Could you check a few things on this model? Use its own coordinates, in mm. A direction names the side the tool comes from. Round coordinates to 2 decimals unless told otherwise and drop trailing zeros. Loops run counter-clockwise (first coordinate to the right, second up) from the corner with the lowest first, then second, coordinate; pieces in that order, holes last. Notation, with made-up numbers: (-26.75, 51) - (-17.75, 51) arc R20 ccw to (-17.75, 67) - close; hole circle Ø8 at (56.25, -7.75). An arc over 180 degrees is marked (long way). Answer as CSV lines item,"result". Start each with the question number.
1) Which directions (+Z, -Z, +X, -X, +Y, -Y) give clear straight access to the entire face, cutting with the end or side of a thin tool? Please do faces 4 (the face through (-4.2, -2.7, -1)), 5 (the face through (0, 1, -6)), 6 (the face through (0, 1, 5)).
2) I'm going to push flat-ended pins straight in: pin 1 Ø6 at (x, z) = (-0.5, 0.5) entering from -Y; pin 2 Ø4 at (y, z) = (-3.5, -0.5) entering from -X; pin 3 Ø5 at (x, z) = (0.5, -3.5) entering from -Y. Where does each tip first touch, or does it pass through?
3) We'd pull the mould along Y, two halves only. Please class faces 1 (the face through (2.3, -2.7, -1)), 2 (the face through (0, 2, -1)), 3 (the face through (0, 0, -1)): pulls with the +Y half, pulls with the -Y half, needs draft (parallel to the pull), parting line crosses it, or undercut.
4) Please list where these lines run through material, in increasing order: line 1 along Z through (x, y) = (3.75, 1); line 2 along X through (y, z) = (0.5, 4.5); line 3 along Y through (x, z) = (-8, 5.5).
5) Suppose I cut it at D-D, the plane z = -1. Write out the boundary of the cut face in (x, y), then the cut area to 3 significant figures.
6) Suppose I cut it at B-B, the plane z = 4. Write out the boundary of the cut face in (x, y).
7) Suppose I cut it at C-C, the plane y = -3. Write out the boundary of the cut face in (x, z), then the cut area to 3 significant figures.
8) Suppose I cut it at A-A, the plane x = 3.25. Write out the boundary of the cut face in (y, z), then the cut area to 3 significant figures.
```python
from build123d import *

# Parameters (mm, degrees)
SKETCH1_W           = 19.9
SKETCH1_H           = 12
BOSS_EXTRUDE1_DEPTH = 2
SKETCH2_W           = 11.8
SKETCH2_H           = 5
CUT_EXTRUDE1_DEPTH  = 3
CHAMFER1_SIZE       = 1.25
SKETCH3_R           = 0.95
BOSS_EXTRUDE2_DEPTH = 5.6
CHAMFER2_SIZE       = 0.2


with BuildPart() as part:
    # Sketch1 → Boss-Extrude1 (new body)
    with BuildSketch(Plane(origin=(0, 0, 0), x_dir=(1, 0, 0), z_dir=(0, 1, 0))):
        Rectangle(SKETCH1_W, SKETCH1_H)
    extrude(amount=BOSS_EXTRUDE1_DEPTH)

    # Sketch2 → Cut-Extrude1 (cut, through all)
    with BuildSketch(Plane(origin=(0, 2, 0), x_dir=(1, 0, 0), z_dir=(0, 1, 0))):
        with Locations((0, -2.5)):
            Rectangle(SKETCH2_W, SKETCH2_H)
    extrude(amount=-CUT_EXTRUDE1_DEPTH, mode=Mode.SUBTRACT)

    # Chamfer1
    chamfer1_edges = [part.edges().sort_by_distance(p)[0] for p in [
        (-9.95, 2, 0),
        (9.95, 2, 0),
    ]]
    chamfer(chamfer1_edges, length=CHAMFER1_SIZE)

    # Sketch3 → Boss-Extrude2 (add)
    with BuildSketch(Plane.XZ):
        with Locations((-3.25, -1)):
            Circle(SKETCH3_R)
        with Locations((3.25, -1)):
            Circle(SKETCH3_R)
    extrude(amount=BOSS_EXTRUDE2_DEPTH)

    # Chamfer2
    chamfer2_edges = [part.edges().sort_by_distance(p)[0] for p in [
        (-4.2, -5.6, -1),
        (2.3, -5.6, -1),
    ]]
    chamfer(chamfer2_edges, length=CHAMFER2_SIZE)


solid = part.part
```
Filled sheet:
1,face 4,"-Y"
1,face 5,"-Z, +X, -X, +Y, -Y"
1,face 6,"+Y, -Y"
2,pin 1,"y = -5.6"
2,pin 2,"x = -4.2"
2,pin 3,"y = 0"
3,face 1,"needs draft"
3,face 2,"pulls with the +Y half"
3,face 3,"pulls with the -Y half"
4,line 1,"-6 to 0, 5 to 6"
4,line 2,"-9.95 to -5.9, 5.9 to 9.95"
4,line 3,"0 to 2"
5,outline,"(-9.95, 0) - (-4.2, 0) - (-4.2, -5.4) - (-4, -5.6) - (-2.5, -5.6) - (-2.3, -5.4) - (-2.3, 0) - (2.3, 0) - (2.3, -5.4) - (2.5, -5.6) - (4, -5.6) - (4.2, -5.4) - (4.2, 0) - (9.95, 0) - (9.95, 0.75) - (8.7, 2) - (-8.7, 2) - (-9.95, 0.75) - close"
5,area,"59.4 mm²"
6,outline,"(-9.95, 0) - (-5.9, 0) - (-5.9, 2) - (-8.7, 2) - (-9.95, 0.75) - close; (5.9, 0) - (9.95, 0) - (9.95, 0.75) - (8.7, 2) - (5.9, 2) - close"
7,outline,"circle Ø1.9 at (-3.25, -1); circle Ø1.9 at (3.25, -1)"
7,area,"5.67 mm²"
8,outline,"(-5.6, -1.75) - (-5.4, -1.95) - (0, -1.95) - (0, -6) - (2, -6) - (2, 0) - (0, 0) - (0, -0.05) - (-5.4, -0.05) - (-5.6, -0.25) - close; (0, 5) - (2, 5) - (2, 6) - (0, 6) - close"
8,area,"24.6 mm²"
